Geometry check sheet. Reference: the model listing, model coordinates, mm. Face numbers are marked on the shaded views. Round coordinates to 2 decimals unless told otherwise and drop trailing zeros. Write each loop counter-clockwise with the first axis right and the second up, starting at its lowest first coordinate (ties: lowest second). Pieces come first, ordered by that corner, then holes. Notation, with made-up numbers: M 63.5,8 L 96.5,8 A25 cw 96.5,33 Z; hole C 44,39 d1. An arc over 180 degrees is marked long. Use a Markdown table: item, result.
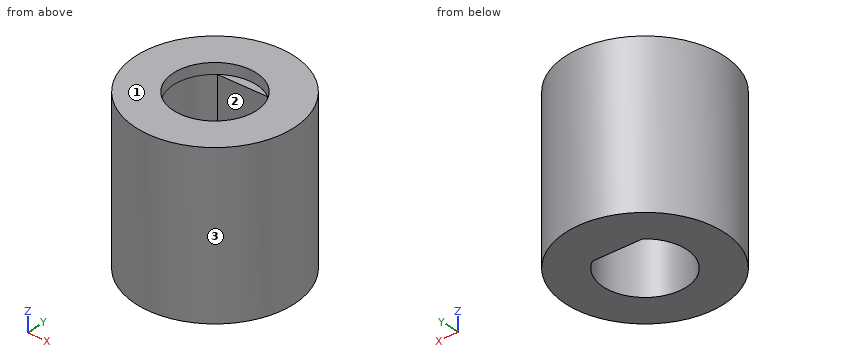
```python
from build123d import *

# Parameters (mm, degrees)
SKETCH1_R           = 4.7625
BOSS_EXTRUDE1_DEPTH = 9
SKETCH2_R           = 4.7625
SKETCH2_R_2         = 2.5
BOSS_EXTRUDE2_DEPTH = 0.652


with BuildPart() as part:
    # Sketch1 → Boss-Extrude1 (new body)
    with BuildSketch(Plane.XY):
        Circle(SKETCH1_R)
        with BuildLine():
            Line((-1.5, 2), (1.5, 2))
            ThreePointArc((1.5, 2), (0, -2.5), (-1.5, 2))
        make_face(mode=Mode.SUBTRACT)
    extrude(amount=BOSS_EXTRUDE1_DEPTH)

    # Sketch2 → Boss-Extrude2 (add)
    with BuildSketch(Plane.XY.offset(9)):
        Circle(SKETCH2_R)
        with Locations(Location((0, 0, 0), (0, 0, 126.869897646))):
            Circle(SKETCH2_R_2, mode=Mode.SUBTRACT)
    extrude(amount=BOSS_EXTRUDE2_DEPTH)


solid = part.part
```
Item 1: Cross-section at C-C, the plane z = 2.5. Record the cut outline in (x, y) (1 decimal).
Outcome:
| item | result |
|---|---|
| outline | C 0,0 d9.5; hole M -1.5,2 A2.5 ccw long 1.5,2 Z |
Item 2: Cross-section at D-D, the plane x = -2. Record the cut outline in (y, z), and give its area (3 significant figures).
Outcome:
| item | result |
|---|---|
| outline | M -4.32,0 L -1.5,0 L -1.5,9.65 L -4.32,9.65 Z; M 1.5,0 L 4.32,0 L 4.32,9.65 L 1.5,9.65 Z |
| area | 54.5 mm2 |
Item 3: Mould release check, pull along Y, two halves, no side actions. Record for the marked faces 1, 2 and 3: +Y half, -Y half, draft (parallel to the pull), parting line (faces both ways), or undercut.
Outcome:
| item | result |
|---|---|
| face 1 | draft |
| face 2 | undercut |
| face 3 | parting line |
Item 4: Go/stop test with a flat-tipped pin: pin 1 (1 mm diameter, centred on x = 2, z = 6, fed in from +Y). Record where the tip stops, or that it passes through.
Outcome:
| item | result |
|---|---|
| pin 1 | stops at y = 4.52 |
Item 5: Cross-section at B-B, the plane x = -0.75. Record the cut outline in (y, z).
Outcome:
| item | result |
|---|---|
| outline | M -4.7,0 L -2.38,0 L -2.38,9.65 L -4.7,9.65 Z; M 2,0 L 4.7,0 L 4.7,9.65 L 2.38,9.65 L 2.38,9 L 2,9 Z |
Item 6: Cross-section at A-A, the plane y = 0. Record the cut outline in (x, z).
Outcome:
| item | result |
|---|---|
| outline | M -4.76,0 L -2.5,0 L -2.5,9.65 L -4.76,9.65 Z; M 2.5,0 L 4.76,0 L 4.76,9.65 L 2.5,9.65 Z |
Item 7: Material ranges on line 1 along Y through (x, z) = (0, 6.5); line 2 along Y through (x, z) = (0, 9.5); line 3 along X through (y, z) = (-1, 6), recorded low to high. Write a range as from..to.
Outcome:
| item | result |
|---|---|
| line 1 | y = -4.76..-2.5, 2..4.76 |
| line 2 | y = -4.76..-2.5, 2.5..4.76 |
| line 3 | x = -4.66..-2.29, 2.29..4.66 |
